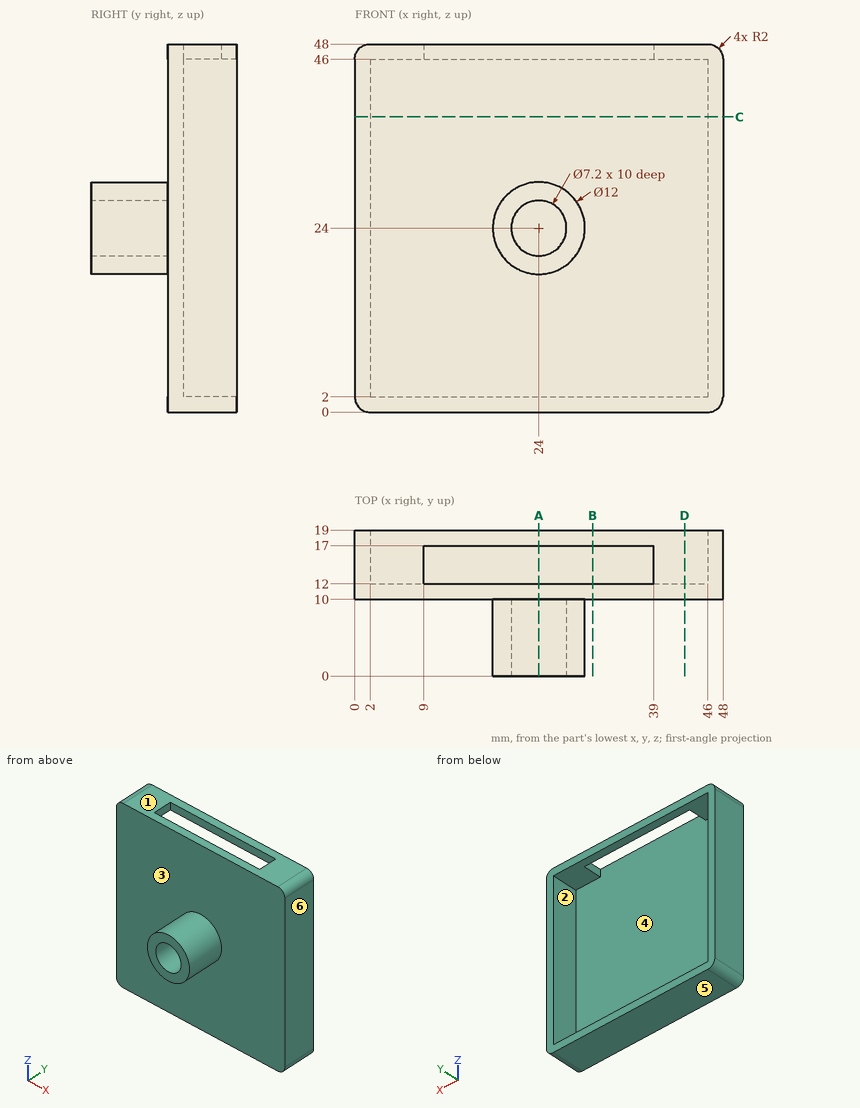
Here's the drawing with two shaded views (mm, measured from the low corner). I have some questions. A direction names the side the tool comes from. Coordinates: 2 decimals unless noted, no trailing zeros. Order: outer loops, then holes, each group sorted by start corner. A loop starts at its lowest first (then second) coordinate and runs counter-clockwise, first axis right, second up. Notation, with made-up numbers: (17, -32.75) -> (57, -32.75) arc R16 ccw to (57, -6.75) -> close; hole circle Ø9 at (46.25, 89). An arc over 180 degrees is marked (long way). One line per question, with ' | ' between items.
Q1. Thinking about a two-plate mould opening in Z: for the marked faces 4, 5 and 6, which applies, pulls with the +Z half, pulls with the -Z half, needs draft (parallel to the pull), parting line crosses it, or undercut?
Return value:
face 4: undercut | face 5: pulls with the -Z half | face 6: needs draft
Q2. Imagine slicing it at A-A on x = 24. Please give me the cut outline in (y, z).
Return value:
outline: (0, 18) -> (10, 18) -> (10, 0) -> (19, 0) -> (19, 2) -> (12, 2) -> (12, 48) -> (10, 48) -> (10, 30) -> (0, 30) -> (0, 27.6) -> (10, 27.6) -> (10, 20.4) -> (0, 20.4) -> close; (17, 46) -> (19, 46) -> (19, 48) -> (17, 48) -> close
Q3. Imagine slicing it at B-B on x = 31. Please give me the cut outline in (y, z), and give its area (3 significant figures).
Return value:
outline: (10, 0) -> (19, 0) -> (19, 2) -> (12, 2) -> (12, 48) -> (10, 48) -> close; (17, 46) -> (19, 46) -> (19, 48) -> (17, 48) -> close | area: 114 mm²
Q4. Imagine slicing it at D-D on x = 43. Please give me the cut outline in (y, z), and give its area (3 significant figures).
Return value:
outline: (10, 0) -> (19, 0) -> (19, 2) -> (12, 2) -> (12, 46) -> (19, 46) -> (19, 48) -> (10, 48) -> close | area: 124 mm²
Q5. If I drill on L1, parallel to X at y = 18, z = 38; L2, parallel to X at y = 3.5, z = 24; L3, parallel to Y at x = 9.5, z = 40, over which ranges is the centre line in solid material (lowest first)?
Return value:
L1: 0 to 2, 46 to 48 | L2: 18 to 20.4, 27.6 to 30 | L3: 10 to 12
Q6. I'm going to push flat-ended pins straight in: P1, Ø8, axis at x = 24.5, z = 23, coming from the -Y side; P2, Ø1.6, axis at x = 28.5, z = 47.5, coming from the -Y side; P3, Ø1, axis at x = 37.5, z = 31, coming from the +Y side; P4, Ø1, axis at y = 13.5, z = 47, coming from the -X side. Where does each tip first touch, or does it pass through?
Return value:
P1: y = 0 | P2: y = 10 | P3: y = 12 | P4: x = 0.06
Q7. On a 3-axis mill with a long thin cutter (end or side, diameter ignored), from which of +Z, -Z, +X, -X, +Y, -Y can I reach the whole of each face in a straight line? I mean the marked faces 1, 2 and 3. Say none if no direction works.
Return value:
face 1: +Z, +X, -X, +Y, -Y | face 2: +Y | face 3: -Y
Q8. Imagine slicing it at C-C on z = 38.5. Please give me the cut outline in (x, y).
Return value:
outline: (0, 10) -> (48, 10) -> (48, 19) -> (46, 19) -> (46, 12) -> (2, 12) -> (2, 19) -> (0, 19) -> close
